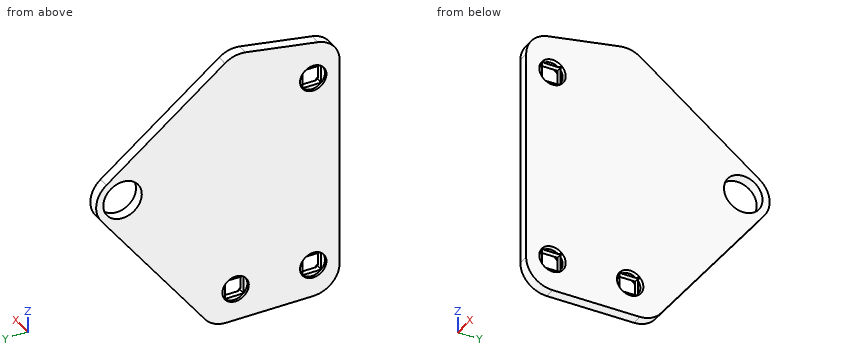
```python
from build123d import *

# Parameters (mm, degrees)
SKETCH1_R           = 3.65
SKETCH1_W           = 3.5
SKETCH1_H           = 3.5
BOSS_EXTRUDE1_DEPTH = 2
SKETCH3_R           = 2.5
CUT_EXTRUDE1_DEPTH  = 0.5
CUT_EXTRUDE1_TAPER  = 30
SKETCH5_R           = 2.5
CUT_EXTRUDE2_DEPTH  = 0.5


with BuildPart() as part:
    # Sketch1 → Boss-Extrude1 (new body)
    with BuildSketch(Plane(origin=(0, 0, 0), x_dir=(0, 0, -1), z_dir=(1, 0, 0))):
        with BuildLine():
            Line((-20.402250922, 0), (20.402250922, 0))
            ThreePointArc((20.402250922, 0), (23.937784828, 1.464466094), (25.402250922, 5))
            Line((25.402250922, 5), (25.402250922, 21.50709196))
            ThreePointArc((25.402250922, 21.50709196), (24.87692273, 23.738081025), (23.411326038, 25.50026951))
            Line((23.411326038, 25.50026951), (-2.635195634, 45.127731407))
            ThreePointArc((-2.635195634, 45.127731407), (-6.321071977, 46.088536103), (-9.61416456, 44.174281334))
            Line((-9.61416456, 44.174281334), (-26.788641191, 21.74435991))
            ThreePointArc((-26.788641191, 21.74435991), (-27.676067974, 19.890565251), (-27.742786146, 17.836391544))
            Line((-27.742786146, 17.836391544), (-25.326289687, 4.131759112))
            ThreePointArc((-25.326289687, 4.131759112), (-23.61618897, 1.169777784), (-20.402250922, 0))
        make_face()
        with Locations((-5.64427075, 41.134553857)):
            Circle(SKETCH1_R, mode=Mode.SUBTRACT)
        with Locations((-18.377749078, 5)):
            Rectangle(SKETCH1_W, SKETCH1_H, mode=Mode.SUBTRACT)
        with Locations((19.182250922, 5)):
            Rectangle(SKETCH1_W, SKETCH1_H, mode=Mode.SUBTRACT)
        with Locations((19.182250922, 19.71162529)):
            Rectangle(SKETCH1_W, SKETCH1_H, mode=Mode.SUBTRACT)
    extrude(amount=BOSS_EXTRUDE1_DEPTH)

    # Sketch3 → Cut-Extrude1 (cut)
    with BuildSketch(Plane(origin=(2, 0, 0), x_dir=(0, 0, -1), z_dir=(1, 0, 0))):
        with Locations((-18.377749078, 5)):
            Circle(SKETCH3_R)
        with Locations((19.182250922, 5)):
            Circle(SKETCH3_R)
        with Locations((19.182250922, 19.712)):
            Circle(SKETCH3_R)
    extrude(amount=-CUT_EXTRUDE1_DEPTH, taper=CUT_EXTRUDE1_TAPER, mode=Mode.SUBTRACT)

    # Sketch5 → Cut-Extrude2 (cut)
    with BuildSketch(Plane.ZY):
        with Locations((-19.182250922, 5)):
            Circle(SKETCH5_R)
        with Locations((-19.182250922, 19.71162529)):
            Circle(SKETCH5_R)
        with Locations((18.377749078, 5)):
            Circle(SKETCH5_R)
    extrude(amount=-CUT_EXTRUDE2_DEPTH, mode=Mode.SUBTRACT)


solid = part.part
```
Part model, mm, in its own coordinate system. Give positions to 0.01 mm unless a question says otherwise; leave off trailing zeros. Loops run counter-clockwise (first coordinate to the right, second up) from the corner with the lowest first, then second, coordinate; pieces in that order, holes last. Notation, with made-up numbers: M 35.25,-27.5 L 82.25,-27.5 A13 ccw 82.25,-21.5 Z; hole C 7,-17 d1. An arc over 180 degrees is marked long. Return JSON: item names as keys, results as strings.
1) Drill centre lines: line 1 (Y direction, x = 1.75, z = -17.5); line 2 (Z direction, x = 1.85, y = 4); line 3 (Z direction, x = 1.85, y = 19). Where is each one in solid material? Low to high.
Calculated:
{"line 1": "y = 0 to 3.25, 6.75 to 17.96, 21.46 to 29.95", "line 2": "z = -25.3 to -21.38, -16.99 to 16.18, 20.57 to 25.3", "line 3": "z = -25.4 to -21.49, -16.88 to 27.81"}
2) Flat gauge pins, fed straight in: pin 1 Ø0.5 at (y, z) = (5, -21) entering from +X; pin 2 Ø1.2 at (x, z) = (1, -19.5) entering from +Y; pin 3 Ø1 at (y, z) = (21, -19.5) entering from -X. Where does each tip first touch, or does it go through?
Calculated:
{"pin 1": "stops at x = 1.5", "pin 2": "stops at y = 28.9", "pin 3": "stops at x = 0.5"}
3) Saw through at B-B, the plane z = -6. List the corners of the cut face in (x, y), then the cut area to 3 significant figures.
Calculated:
{"outline": "M 0,0 L 2,0 L 2,38.62 L 0,38.62 Z", "area": "77.2 mm2"}
4) Saw through at A-A, the plane y = 39. List the corners of the cut face in (x, z).
Calculated:
{"outline": "M 0,-5.5 L 2,-5.5 L 2,2.68 L 0,2.68 Z; M 0,8.61 L 2,8.61 L 2,13.58 L 0,13.58 Z"}
5) Saw through at C-C, the plane y = 28. List the corners of the cut face in (x, z).
Calculated:
{"outline": "M 0,-20.09 L 2,-20.09 L 2,22 L 0,22 Z"}
